```python
from build123d import *

# Parameters (mm, degrees)
BOSS_EXTRUDE3_DEPTH     = 3
SKETCH14_W              = 3
SKETCH14_H              = 37
BOSS_EXTRUDE8_DEPTH     = 3
SKETCH15_R              = 2
BOSS_EXTRUDE9_DEPTH     = 10
BOSS_EXTRUDE10_START    = -3
SKETCH16_R              = 2
BOSS_EXTRUDE10_DEPTH    = 3
CUT_EXTRUDE6_DEPTH      = 36.65196348
CUT_EXTRUDE6_DEPTH_BACK = 36.65196348
SKETCH18_W              = 39.290830544
SKETCH18_H              = 5
FILLET1_R               = 4
SKETCH19_R              = 1.25
SKETCH19_W              = 10
SKETCH19_H              = 27
CUT_EXTRUDE7_DEPTH      = 10


with BuildPart() as part:
    # Sketch1 → Boss-Extrude3 (new body)
    with BuildSketch(Plane(origin=(0, 0, 0), x_dir=(1, 0, 0), z_dir=(0, 1, 0))):
        Polygon((-14, -6.25), (-14, 13.75), (-14, 22.25), (14, 22.25), (14, 13.75), (14, -6.25), (14, -14.75), (-14, -14.75), align=None)
    extrude(amount=BOSS_EXTRUDE3_DEPTH)

    # Sketch14 → Boss-Extrude8 (add)
    with BuildSketch(Plane.XZ):
        with Locations((-15.5, -3.75)):
            Rectangle(SKETCH14_W, SKETCH14_H)
        with Locations((15.5, -3.75)):
            Rectangle(SKETCH14_W, SKETCH14_H)
    extrude(amount=-BOSS_EXTRUDE8_DEPTH)

    # Sketch15 → Boss-Extrude9 (add)
    # profile 1 of 2: a face of its own
    with BuildSketch(Plane(origin=(0, 0, 0), x_dir=(1, 0, 0), z_dir=(0, 1, 0))):
        with BuildLine():
            Line((-25.3034482, 6.555964573), (-17, 22.25))
            Line((-17, 22.25), (-14, 22.25))
            Line((-14, 22.25), (-14, -14.75))
            Line((-14, -14.75), (-17, -14.75))
            Line((-17, -14.75), (-25.3034482, 0.944035427))
            ThreePointArc((-25.3034482, 0.944035427), (-26, 3.75), (-25.3034482, 6.555964573))
        make_face()
        with Locations(Location((-20, 3.75, 0), (0, 0, 270))):
            Circle(SKETCH15_R, mode=Mode.SUBTRACT)
    # profile 2 of 2: a face of its own
    with BuildSketch(Plane(origin=(0, 0, 0), x_dir=(1, 0, 0), z_dir=(0, 1, 0))):
        with BuildLine():
            Line((17, 22.25), (25.3034482, 6.555964573))
            ThreePointArc((25.3034482, 6.555964573), (26, 3.75), (25.3034482, 0.944035427))
            Line((25.3034482, 0.944035427), (17, -14.75))
            Line((17, -14.75), (14, -14.75))
            Line((14, -14.75), (14, 22.25))
            Line((14, 22.25), (17, 22.25))
        make_face()
        with Locations(Location((20, 3.75, 0), (0, 0, 270))):
            Circle(SKETCH15_R, mode=Mode.SUBTRACT)
    extrude(amount=BOSS_EXTRUDE9_DEPTH)

    # Sketch16 → Boss-Extrude10 (add)
    with BuildSketch(Plane(origin=(0, 10, 0), x_dir=(1, 0, 0), z_dir=(0, 1, 0)).offset(BOSS_EXTRUDE10_START)):
        with Locations(Location((20, 3.75, 0), (0, 0, 270))):
            Circle(SKETCH16_R)
        with Locations(Location((-20, 3.75, 0), (0, 0, 270))):
            Circle(SKETCH16_R)
    extrude(amount=BOSS_EXTRUDE10_DEPTH)

    # Sketch18 → Cut-Extrude6 (cut, two sides: drawn at the far end of the back side and taken through both)
    with BuildSketch(Plane.XZ.offset(-CUT_EXTRUDE6_DEPTH_BACK)):
        with Locations((0, 12.25)):
            Rectangle(SKETCH18_W, SKETCH18_H)
    extrude(amount=CUT_EXTRUDE6_DEPTH + CUT_EXTRUDE6_DEPTH_BACK, mode=Mode.SUBTRACT)

    # Fillet1
    fillet1_edges = [part.edges().sort_by_distance(p)[0] for p in [
        (19.645415272, 5, 9.75),
        (-19.645415272, 5, 9.75),
        (-17, 5, -22.25),
        (17, 5, -22.25),
    ]]
    fillet(fillet1_edges, radius=FILLET1_R)

    # Sketch19 → Cut-Extrude7 (cut)
    with BuildSketch(Plane(origin=(0, 3, 0), x_dir=(1, 0, 0), z_dir=(0, 1, 0))):
        with Locations(Location((-6.8, 14.55, 0), (0, 0, 270))):
            Circle(SKETCH19_R)
        with Locations(Location((6.8, 14.55, 0), (0, 0, 270))):
            Circle(SKETCH19_R)
        with Locations((0, 7.5)):
            Rectangle(SKETCH19_W, SKETCH19_H)
    extrude(amount=-CUT_EXTRUDE7_DEPTH, mode=Mode.SUBTRACT)


solid = part.part
```
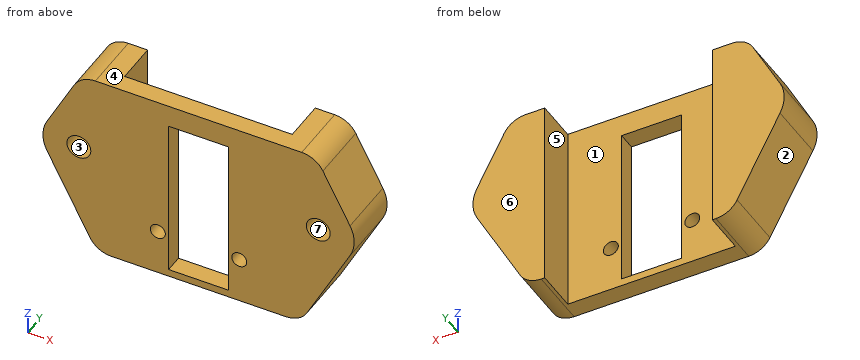
Could you check a few things on this model? Use its own coordinates, in mm. Face numbers are marked on the shaded views. A direction names the side the tool comes from. Coordinates: 2 decimals unless noted, no trailing zeros. Loops run counter-clockwise (first coordinate to the right, second up) from the corner with the lowest first, then second, coordinate; pieces in that order, holes last. Notation, with made-up numbers: M 59.5,-40 L 102.5,-40 A12 ccw 102.5,-36 Z; hole C -16.5,54 d7. An arc over 180 degrees is marked long. Put each result on its own line as item: value. Start each with the question number.
(1) I need wall thicknesses on line 1 (Z direction, x = 1.5, y = 2.25); line 2 (X direction, y = 1.6, z = -14.55); line 3 (Y direction, x = -8, z = -2). Which ranges of each line are inside material? Lowest first, please. Write a range as from..to.
(2) Will these pins go through, and if not, where does the flat tip stop? P1, Ø5, axis at y = 8.5, z = 0.5, coming from the -X side; P2, Ø1.2, axis at x = -19.5, z = -4, coming from the -Y side; P3, Ø3.5, axis at y = 6.5, z = -13, coming from the -X side.
(3) Suppose I cut it at A-A on y = 5. Please give me the cut outline in (x, z), then the cut area to 3 significant figures.
(4) Suppose I cut it at C-C on z = 5. Please give me the cut outline in (x, y).
(5) For the marked faces 5, 6 and 7, which set-ups out of +Z, -Z, +X, -X, +Y, -Y let a thin tool reach every point of the face, with its end or its side?
(6) Thinking about a two-plate mould opening in X: for the marked faces 1, 2, 3 and 4, which applies, pulls with the +X half, pulls with the -X half, needs draft (parallel to the pull), parting line crosses it, or undercut?
(7) Suppose I cut it at D-D on y = 2.5. Please give me the cut outline in (x, z).
(8) Suppose I cut it at B-B on x = 6.8. Please give me the cut outline in (y, z), then the cut area to 3 significant figures.
Solutions:
1. line 1: z = -22.25..-21, 6..9.75
1. line 2: x = -21.07..-8.05, -5.55..-5, 5..5.55, 8.05..21.07
1. line 3: y = 0..3
2. P1: stops at x = -25.74
2. P2: stops at y = 7
2. P3: stops at x = -22.82
3. outline: M -25.3,-6.56 L -18.13,-20.12 A4 ccw -14.59,-22.25 L -14,-22.25 L -14,9.75 L -17.24,9.75 A4 ccw -20.77,7.62 L -25.3,-0.94 A6 ccw Z; M 14,-22.25 L 14.59,-22.25 A4 ccw 18.13,-20.12 L 25.3,-6.56 A6 ccw 25.3,-0.94 L 20.77,7.62 A4 ccw 17.24,9.75 L 14,9.75 Z; hole C -20,-3.75 d4; hole C 20,-3.75 d4
3. area: 509 mm2
4. outline: M -22.16,0 L -5,0 L -5,3 L -14,3 L -14,10 L -22.16,10 Z; M 5,0 L 22.16,0 L 22.16,10 L 14,10 L 14,3 L 5,3 Z
5. face 5: +Z, -Z, +Y
5. face 6: +Z, -Z, +X, -X, +Y
5. face 7: -Y
6. face 1: undercut
6. face 2: pulls with the -X half
6. face 3: undercut
6. face 4: needs draft
7. outline: M -25.3,-6.56 L -18.13,-20.12 A4 ccw -14.59,-22.25 L 14.59,-22.25 A4 ccw 18.13,-20.12 L 25.3,-6.56 A6 ccw 25.3,-0.94 L 20.77,7.62 A4 ccw 17.24,9.75 L -17.24,9.75 A4 ccw -20.77,7.62 L -25.3,-0.94 A6 ccw Z; hole C -20,-3.75 d4; hole C -6.8,-14.55 d2.5; hole M -5,-21 L 5,-21 L 5,6 L -5,6 Z; hole C 6.8,-14.55 d2.5; hole C 20,-3.75 d4
8. outline: M 0,-22.25 L 3,-22.25 L 3,-15.8 L 0,-15.8 Z; M 0,-13.3 L 3,-13.3 L 3,9.75 L 0,9.75 Z
8. area: 88.5 mm2
